The model under review builds one solid part; all positions refer to its coordinate system, in mm. Round coordinates to 2 decimals unless told otherwise and drop trailing zeros. Order: outer loops, then holes, each group sorted by start corner. A loop starts at its lowest first (then second) coordinate and runs counter-clockwise, first axis right, second up.
from build123d import *

# Parameters (mm, degrees)
SKETCH_1_R          = 70
SKETCH_1_R_2        = 56
EXTRUDE_1_DEPTH     = 2
SKETCH_2_R          = 1.5
CUT_EXTRUDE_1_DEPTH = 3
CHAMFER_1_SIZE      = 1.5


with BuildPart() as part:
    # 草图1 → 凸台-拉伸1 (new body)
    with BuildSketch(Plane(origin=(0, 0, 0), x_dir=(1, 0, 0), z_dir=(0, 1, 0))):
        with Locations(Location((0, 0, 0), (0, 0, 270))):
            Circle(SKETCH_1_R)
        with Locations(Location((0, 0, 0), (0, 0, 270))):
            Circle(SKETCH_1_R_2, mode=Mode.SUBTRACT)
    extrude(amount=EXTRUDE_1_DEPTH)

    # 草图2 → 切除-拉伸1 (cut)
    with BuildSketch(Plane(origin=(0, 2, 0), x_dir=(1, 0, 0), z_dir=(0, 1, 0))):
        with Locations(Location((42.423982239, 50.558933246, 0), (0, 0, 270))):
            Circle(SKETCH_2_R)
        with Locations(Location((50.558933246, 42.423982239, 0), (0, 0, 270))):
            Circle(SKETCH_2_R)
        with Locations(Location((-50.558933246, 42.423982239, 0), (0, 0, 270))):
            Circle(SKETCH_2_R)
        with Locations(Location((-42.423982239, 50.558933246, 0), (0, 0, 270))):
            Circle(SKETCH_2_R)
        with Locations(Location((-50.558933246, -42.423982239, 0), (0, 0, 270))):
            Circle(SKETCH_2_R)
        with Locations(Location((-42.423982239, -50.558933246, 0), (0, 0, 270))):
            Circle(SKETCH_2_R)
        with Locations(Location((22.573329459, -62.019712972, 0), (0, 0, 270))):
            Circle(SKETCH_2_R)
        with Locations(Location((62.019712972, -22.573329459, 0), (0, 0, 270))):
            Circle(SKETCH_2_R)
    extrude(amount=-CUT_EXTRUDE_1_DEPTH, mode=Mode.SUBTRACT)

    # 倒角1
    chamfer_1_edges = [part.edges().sort_by_distance(p)[0] for p in [
        (50.558933246, 2, -43.923982239),
        (22.573329459, 2, 60.519712972),
        (-50.558933246, 2, -43.923982239),
        (-42.423982239, 2, -52.058933246),
        (-50.558933246, 2, 40.923982239),
        (-42.423982239, 2, 49.058933246),
        (62.019712972, 2, 21.073329459),
        (42.423982239, 2, -52.058933246),
    ]]
    chamfer(chamfer_1_edges, length=CHAMFER_1_SIZE)


solid = part.part
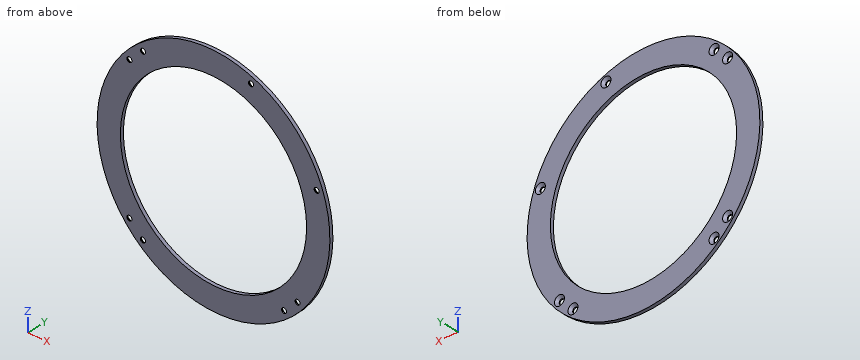
(1) We need section C-C (y = 1.4). Count the separate pieces of the cut face and the enclosed holes in it, and give its area (3 significant figures).
(2) Clearance check with a flat-ended pin moving along its axis: P1, Ø1, axis at x = -53, y = 0.5, coming from the +Z side. State where the tip first meets the part, or that it passes through.
(3) We need section B-B (z = 0). Give the boundary of the cut face in (x, y).
(4) To check wall thickness, follow L1, parallel to X at y = 1.85, z = -43.5; L2, parallel to X at y = 0.75, z = 0; L3, parallel to Z at x = -41, y = 1.8. State the ranges of each line that lie inside material, in increasing order.
(5) We need section A-A (x = 0). Give the boundary of the cut face in (y, z), and give its area (3 significant figures).
Verdict:
1. separate pieces: 1
1. enclosed holes: 9
1. area: 5,400 mm2
2. P1: stops at z = 46.3
3. outline: (-70, 0) - (-56, 0) - (-56, 2) - (-70, 2) - close; (56, 0) - (70, 0) - (70, 2) - (56, 2) - close
4. L1: x = -54.84 to -53.2, -47.92 to -35.27, 35.27 to 47.92, 53.2 to 54.84
4. L2: x = -70 to -56, 56 to 70
4. L3: z = -56.74 to -52.97, -48.15 to -38.14, 38.14 to 48.15, 52.97 to 56.74
5. outline: (0, -70) - (2, -70) - (2, -56) - (0, -56) - close; (0, 56) - (2, 56) - (2, 70) - (0, 70) - close
5. area: 56.0 mm2
